Can you work these out from the model? Positions are in its coordinate system, mm. Face numbers are marked on the shaded views. A direction names the side the tool comes from. Give positions to 0.01 mm unless a question says otherwise; leave off trailing zeros. Write each loop counter-clockwise with the first axis right and the second up, starting at its lowest first coordinate (ties: lowest second). Pieces come first, ordered by that corner, then holes. Notation, with made-up numbers: (-6, 10.25) - (15, 10.25) arc R36 ccw to (15, 46.25) - close; hole circle Ø4 at (16.5, -30.5). An arc over 180 degrees is marked (long way). Return JSON: item names as keys, results as strings. Group by question number.
from build123d import *

# Parameters (mm, degrees)
CROQUIS1_W              = 24
CROQUIS1_H              = 10
SALIENTE_EXTRUIR1_DEPTH = 14.21
CROQUIS2_W              = 17
CROQUIS2_H              = 8.5
CORTAR_EXTRUIR1_DEPTH   = 12
CROQUIS3_R              = 1.6
CORTAR_EXTRUIR2_DEPTH   = 29.335915373
CROQUIS4_R              = 1.55
CORTAR_EXTRUIR3_DEPTH   = 12


with BuildPart() as part:
    # Croquis1 → Saliente-Extruir1 (new body)
    with BuildSketch(Plane.XY):
        Rectangle(CROQUIS1_W, CROQUIS1_H)
    extrude(amount=SALIENTE_EXTRUIR1_DEPTH)

    # Croquis2 → Cortar-Extruir1 (cut)
    with BuildSketch(Plane.XZ.offset(5)):
        with Locations((0, 9.96)):
            Rectangle(CROQUIS2_W, CROQUIS2_H)
    extrude(amount=-CORTAR_EXTRUIR1_DEPTH, mode=Mode.SUBTRACT)

    # Croquis3 → Cortar-Extruir2 (cut, through all)
    with BuildSketch(Plane.ZY.offset(12)):
        with Locations((10.21, 0)):
            Circle(CROQUIS3_R)
    extrude(amount=-CORTAR_EXTRUIR2_DEPTH, mode=Mode.SUBTRACT)

    # Croquis4 → Cortar-Extruir3 (cut)
    with BuildSketch(Plane.XY.offset(5.71)):
        with Locations((-4.5, 0)):
            Circle(CROQUIS4_R)
        with Locations((4.5, 0)):
            Circle(CROQUIS4_R)
    extrude(amount=-CORTAR_EXTRUIR3_DEPTH, mode=Mode.SUBTRACT)


solid = part.part
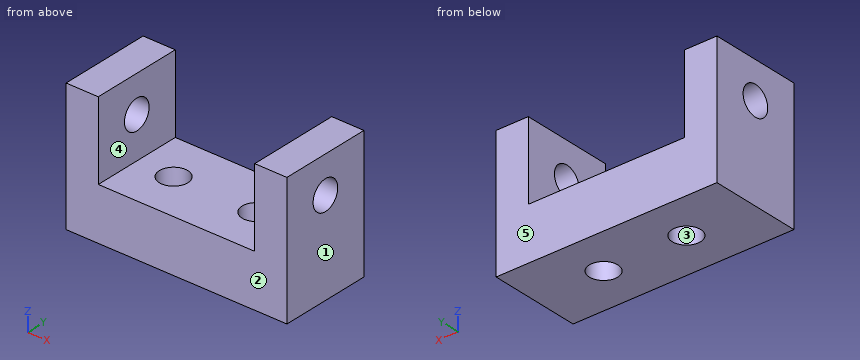
1) I need wall thicknesses on line 1 along Y through (x, z) = (10.1, 10.21); line 2 along X through (y, z) = (-1.75, 11.75); line 3 along Y through (x, z) = (-4.5, 1.4). Which ranges of each line are inside material? Lowest first, please.
2) Imagine slicing it at C-C, the plane z = 10.21. Write out the boundary of the cut face in (x, y), and give its area (3 significant figures).
3) On a 3-axis mill with a long thin cutter (end or side, diameter ignored), from which of +Z, -Z, +X, -X, +Y, -Y can I reach the whole of each face in a straight line? I mean the marked faces 4 and 5. Say none if no direction works.
4) Imagine slicing it at A-A, the plane y = 0. Write out the boundary of the cut face in (x, z).
5) Imagine slicing it at B-B, the plane x = -4.5. Write out the boundary of the cut face in (y, z), and give its area (3 significant figures).
6) We'd pull the mould along Y, two halves only. Please class the marked faces 1, 2 and 3: pulls with the +Y half, pulls with the -Y half, needs draft (parallel to the pull), parting line crosses it, or undercut.
7) Imagine slicing it at D-D, the plane y = 3.5. Write out the boundary of the cut face in (x, z), and give its area (3 significant figures).
8) Will these pins go through, and if not, where does the flat tip stop? pin 1 Ø2 at (x, y) = (2, -3) entering from -Z; pin 2 Ø3 at (x, y) = (4.5, 0) entering from +Z; pin 3 Ø5 at (x, y) = (2, 1) entering from +Z.
Resolved:
{
 "1": {"line 1": "-5 to -1.6, 1.6 to 5", "line 2": "-12 to -8.5, 8.5 to 12", "line 3": "-5 to -1.55, 1.55 to 5"},
 "2": {"outline": "(-12, -5) - (-8.5, -5) - (-8.5, -1.6) - (-12, -1.6) - close; (-12, 1.6) - (-8.5, 1.6) - (-8.5, 5) - (-12, 5) - close; (8.5, -5) - (12, -5) - (12, -1.6) - (8.5, -1.6) - close; (8.5, 1.6) - (12, 1.6) - (12, 5) - (8.5, 5) - close", "area": "47.6 mm^2"},
 "3": {"face 4": "+Z, +Y, -Y", "face 5": "+Z, -Z, +X, -X, +Y"},
 "4": {"outline": "(-12, 0) - (-6.05, 0) - (-6.05, 5.71) - (-8.5, 5.71) - (-8.5, 8.61) - (-12, 8.61) - close; (-12, 11.81) - (-8.5, 11.81) - (-8.5, 14.21) - (-12, 14.21) - close; (-2.95, 0) - (2.95, 0) - (2.95, 5.71) - (-2.95, 5.71) - close; (6.05, 0) - (12, 0) - (12, 8.61) - (8.5, 8.61) - (8.5, 5.71) - (6.05, 5.71) - close; (8.5, 11.81) - (12, 11.81) - (12, 14.21) - (8.5, 14.21) - close"},
 "5": {"outline": "(-5, 0) - (-1.55, 0) - (-1.55, 5.71) - (-5, 5.71) - close; (1.55, 0) - (5, 0) - (5, 5.71) - (1.55, 5.71) - close", "area": "39.4 mm^2"},
 "6": {"face 1": "needs draft", "face 2": "pulls with the -Y half", "face 3": "undercut"},
 "7": {"outline": "(-12, 0) - (12, 0) - (12, 14.21) - (8.5, 14.21) - (8.5, 5.71) - (-8.5, 5.71) - (-8.5, 14.21) - (-12, 14.21) - close", "area": "197 mm^2"},
 "8": {"pin 1": "z = 0", "pin 2": "through", "pin 3": "z = 5.71"}
}
